Here's the drawing with two shaded views (mm, measured from the low corner). I have some questions. A direction names the side the tool comes from. Coordinates: 2 decimals unless noted, no trailing zeros. Write each loop counter-clockwise with the first axis right and the second up, starting at its lowest first coordinate (ties: lowest second). Pieces come first, ordered by that corner, then holes. Notation, with made-up numbers: M 29,-28.75 L 65,-28.75 A28 ccw 65,-6.75 Z; hole C 48,-10 d3. An arc over 180 degrees is marked long. Answer as CSV lines item,"result". Start each with the question number.
Item 1: Suppose I cut it at C-C, the plane z = 17. Write out the boundary of the cut face in (x, y).
Item 2: Suppose I cut it at B-B, the plane y = 29. Write out the boundary of the cut face in (x, z).
Item 3: On a 3-axis mill with a long thin cutter (end or side, diameter ignored), from which of +Z, -Z, +X, -X, +Y, -Y can I reach the whole of each face in a straight line? I mean the marked faces 1, 2 and 3. Say none if no direction works.
Item 4: If I drill on line 1 along Y through (x, z) = (35, 16); line 2 along Z through (x, y) = (60, 5); line 3 along Y through (x, z) = (46.5, 23), over which ranges is the centre line in solid material (lowest first)? Write a range as [from, to].
Item 5: Suppose I cut it at D-D, the plane y = 16. Write out the boundary of the cut face in (x, z).
Item 6: We'd pull the mould along Y, two halves only. Please class the marked faces 4, 5 and 6: +Y half, -Y half, draft (parallel to the pull), parting line (faces both ways), or undercut.
Item 7: Suppose I cut it at A-A, the plane x = 60. Write out the boundary of the cut face in (y, z).
Item 8: I'm going to push flat-ended pins straight in: P1, Ø9.5, axis at y = 23.5, z = 18, coming from the -X side; P2, Ø2, axis at x = 50, z = 20.5, coming from the +Y side; P3, Ø6, axis at y = 23.5, z = 7, coming from the +X side; P4, Ø8.5, axis at x = 60, z = 16, coming from the -Y side. Where does each tip first touch, or does it pass through?
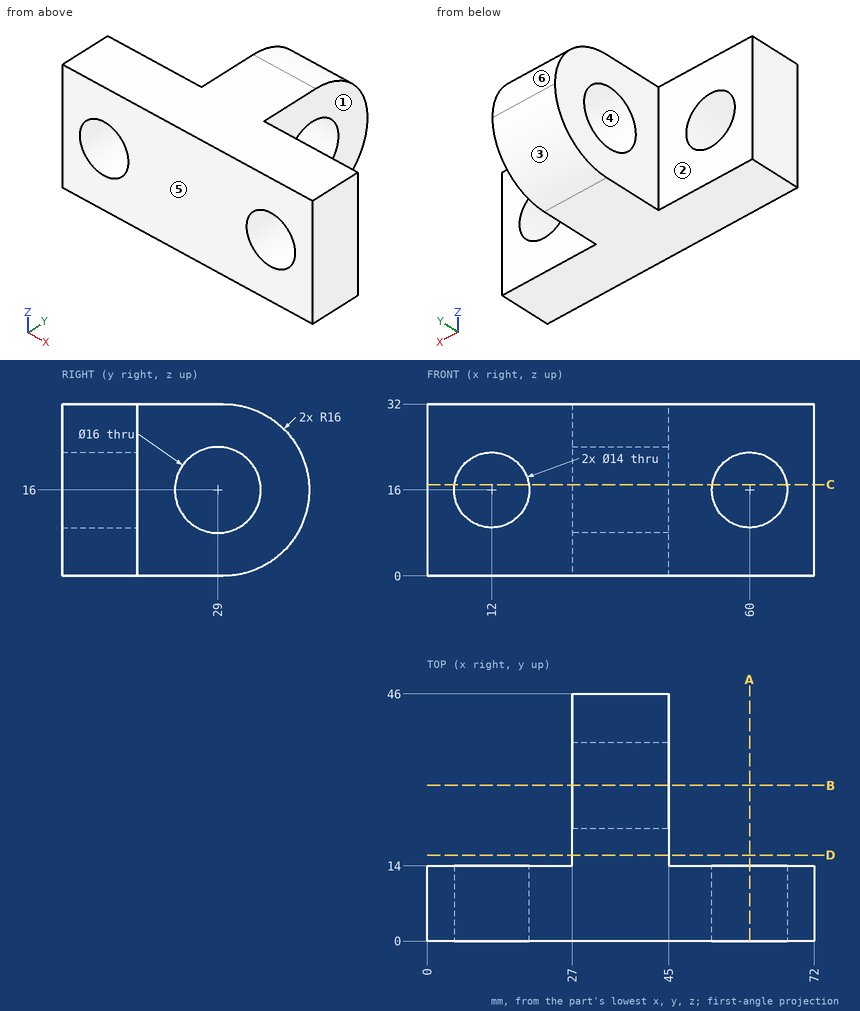
Ans:
1,outline,"M 0,0 L 5.07,0 L 5.07,14 L 0,14 Z; M 18.93,0 L 53.07,0 L 53.07,14 L 45,14 L 45,21.06 L 27,21.06 L 27,14 L 18.93,14 Z; M 27,36.94 L 45,36.94 L 45,45.97 L 27,45.97 Z; M 66.93,0 L 72,0 L 72,14 L 66.93,14 Z"
2,outline,"M 27,0 L 45,0 L 45,8 L 27,8 Z; M 27,24 L 45,24 L 45,32 L 27,32 Z"
3,face 1,"+Z, -Z, +X, +Y"
3,face 2,"+Z, -Z, -X, +Y"
3,face 3,"-Z, +X, -X, +Y"
4,line 1,"y = [0, 21], [37, 46]"
4,line 2,"z = [0, 9], [23, 32]"
4,line 3,"y = [0, 14]"
5,outline,"M 27,0 L 45,0 L 45,32 L 27,32 Z"
6,face 4,"undercut"
6,face 5,"-Y half"
6,face 6,"+Y half"
7,outline,"M 0,0 L 14,0 L 14,9 L 0,9 Z; M 0,23 L 14,23 L 14,32 L 0,32 Z"
8,P1,"stops at x = 27"
8,P2,"stops at y = 14"
8,P3,"stops at x = 45"
8,P4,"passes through"
